```python
from build123d import *

# Parameters (mm, degrees)
F1_DEPTH = 101.6
F2_W     = 25.4
F2_H     = 101.6
F3_DEPTH = 12.7
F4_R     = 25.4
F5_DEPTH = 25.4
F6_DEPTH = 192.786


with BuildPart() as f1:
    # F0 (on Top) → F1 (new body)
    with BuildSketch(Plane.XY):
        Polygon((152.4, 0), (0, 0), (0, -76.2), align=None)
    extrude(amount=F1_DEPTH)

    # F2 (on face) → F3 (cut)
    with BuildSketch(Plane(origin=(30.48, -60.96, 0), x_dir=(0.894427191, 0.4472135955, 0), z_dir=(0.4472135955, -0.894427191, 0))):
        with Locations((54.8223240229, 50.8)):
            Rectangle(F2_W, F2_H)
    extrude(amount=-F3_DEPTH, mode=Mode.SUBTRACT)

    # F4 (on face) → F5 (join)
    with BuildSketch(Plane(origin=(30.48, -60.96, 0), x_dir=(0.894427191, 0.4472135955, 0), z_dir=(0.4472135955, -0.894427191, 0))):
        with Locations((54.8223240229, 50.8)):
            Circle(F4_R)
    extrude(amount=F5_DEPTH)

    # F6 (cut): a face of the model
    f6_faces = [f1.faces().sort_by_distance(p)[0] for p in [
        (90.8738026056, -59.1611620115, 50.8),
    ]]
    extrude(f6_faces, amount=-F6_DEPTH, mode=Mode.SUBTRACT)


solid = f1.part
```
Could you check a few things on this model? Use its own coordinates, in mm. A direction names the side the tool comes from. Coordinates: 2 decimals unless noted, no trailing zeros. Loops run counter-clockwise (first coordinate to the right, second up) from the corner with the lowest first, then second, coordinate; pieces in that order, holes last. Notation, with made-up numbers: M -9.75,44.25 L 35.25,44.25 A25 ccw 35.25,69.25 Z; hole C 4,87 d5. An arc over 180 degrees is marked long. Put each result on its own line as item: value. Start each with the question number.
(1) Suppose I cut it at A-A on z = 31.5. Please give me the cut outline in (x, y) (3 decimals).
(2) For faces 1 (the face through (65.355, -36.522, 86.997)), 2 (the face through (88.074, -25.163, 14.2)), 3 (the face through (74, -25, 87)), which set-ups out of +Z, -Z, +X, -X, +Y, -Y let a thin tool reach every point of the face, with its end or its side?
(3) I need wall thicknesses on line 1 (Z direction, x = 59, y = -38); line 2 (X direction, y = -19, z = 58); line 3 (Z direction, x = 61.5, y = -35). Which ranges of each line are inside material? Lowest first, please. Write a range as from..to.
(4) Suppose I cut it at C-C on x = 22.5. Please give me the cut outline in (y, z).
(5) Thinking about a two-plate mould opening in X: for faces 4 (the face through (74, -25, 15)), 5 (the face through (0, -38, 50)), 6 (the face through (33.6, -59.4, 50.1)), which applies, pulls with the +X half, pulls with the -X half, needs draft (parallel to the pull), parting line crosses it, or undercut?
(6) Suppose I cut it at B-B on z = 11. Please give me the cut outline in (x, y), then the cut area to 3 significant figures.
(7) Suppose I cut it at D-D on y = -28.5. Count the separate pieces of the cut face and the enclosed holes in it, then the cut area to 3 significant figures.
(8) Will these pins go through, and if not, where does the flat tip stop? P1, Ø4, axis at y = -16.5, z = 63.5, coming from the +X side; P2, Ø3, axis at y = -36, z = 47, coming from the -X side; P3, Ø6, axis at x = 68.5, z = 18.5, coming from the -Y side; P4, Ø12, axis at x = 22, z = 28.5, coming from the -Y side.
Solutions:
1. outline: M 0,-76.2 L 64.745,-43.827 L 42.831,0 L 0,0 Z; M 79.755,0 L 94.284,-29.058 L 152.4,0 Z
2. face 1: +Z, -Z, +X
2. face 2: +Z, -Z, -Y
2. face 3: +Z, -Z
3. line 1: z = 0..33.99, 67.61..101.6
3. line 2: x = 0..43.56, 98.03..114.4
3. line 3: z = 0..30.65, 70.95..101.6
4. outline: M -64.95,0 L 0,0 L 0,101.6 L -64.95,101.6 Z
5. face 4: undercut
5. face 5: pulls with the -X half
5. face 6: pulls with the +X half
6. outline: M 0,-76.2 L 68.16,-42.12 L 62.48,-30.76 L 85.19,-19.4 L 90.87,-30.76 L 152.4,0 L 0,0 Z
6. area: 5,480 mm2
7. separate pieces: 3
7. enclosed holes: 0
7. area: 6,450 mm2
8. P1: stops at x = 123.4
8. P2: stops at x = 0
8. P3: stops at y = -43.45
8. P4: stops at y = -68.2
